Geometry: final body of the model. Coordinates: model frame, mm. Face numbers are marked on the shaded views. A direction names the side the tool comes from. Coordinates: 2 decimals unless noted, no trailing zeros. Write each loop counter-clockwise with the first axis right and the second up, starting at its lowest first coordinate (ties: lowest second). Pieces come first, ordered by that corner, then holes. Notation, with made-up numbers: (73, -15.5) -> (111, -15.5) arc R16 ccw to (111, 0.5) -> close; hole circle Ø6 at (37, -31.75). An arc over 180 degrees is marked (long way). One line per item, written item: value.
Autodesk Inventor part; units mm, degrees
ref_plane "Work Plane1" through (29, 0, 0) normal (0, -1, 0) x (1, 0, 0)
ref_plane "YZ Plane" through (0, 0, 0) normal (1, 0, 0) x (0, 1, 0)
ref_plane "XZ Plane" through (0, 0, 0) normal (0, 1, 0) x (-1, 0, 0)
sketch "Skizze1" plane through (0, 0, 0) normal (0, 0, 1) x (1, 0, 0)
  line L0 (-0.5, 0) -> (20, 0)
  line L1 (20, 0) -> (20, 1)
  line L2 (20, 1) -> (1, 1)
  line L3 (1, 1) -> (0.7545, 1)
  line L4 (0.7545, 1) -> (0, 1)
  line L5 (0, 1) -> (0, 1.9)
  line L6 (0, 1.9) -> (-2, 1.9)
  line L7 (-2, 1.9) -> (-2, 0.866)
  line L8 (-2, 0.866) -> (-1, 0.866)
  line L9 (-1, 0.866) -> (-0.5, 0)
  line L10 (-6.4, 0) -> (24.4, 0)
  line L11 (0, -0.38) -> (0, 2.28)
  line L12 (1, 1) -> (0, 1) construction
  dimension "d1" = 19
  dimension "d2" = 0.2455
  dimension "d3" = 2
  dimension "d4" = 1
  dimension "d5" = 60
  dimension "d6" = 2
  dimension "d7" = 2
  dimension "d8" = 1.7321
  dimension "d9" = 3.8
  dimension "d26" = 20
revolve "Körper" add sketch "Skizze1" angle 360 about axis through (-0.5, 0, 0) along (1, 0, 0)
sketch "Skizze2" plane through (-2, 0, 0) normal (-1, 0, 0) x (0, 0, 1)
  circle A0 centre (0, 0) radius 0.866
  line L0 (0, -2.66) -> (0, 2.66)
  line L1 (-2.66, 0) -> (2.66, 0)
  line L2 (0.866, 0) -> (0.433, -0.75)
  line L3 (0.433, -0.75) -> (-0.433, -0.75)
  line L4 (-0.433, -0.75) -> (-0.866, 0)
  line L5 (-0.866, 0) -> (-0.433, 0.75)
  line L6 (-0.433, 0.75) -> (0.433, 0.75)
  line L7 (0.433, 0.75) -> (0.866, 0)
extrude "Loch" add sketch "Skizze2" against normal up to next contours L7 A0 | A0 L2 | L6 L0 A0 | A0 L0 L3 | L0 L6 A0 | A0 L3 L0 | L4 A0 | A0 L5
fillet "Rundung1" radius 0.2 1 edges at (-2, -1.9, 0)
thread "Gewinde"
chamfer "Fase1" distance 0.2454 distance2 0.2454 1 edges at (20, -1, 0) measured on face at (20, -0.4443, -0.4503)
ref_plane "Work Plane1" through (29, 0, 0) normal (0, -1, 0) x (1, 0, 0)
fillet "Fillet2" radius 0.1 1 edges at (0, -1, 0)
equation "\"d1\" = GEL"
equation "\"d3\" = KOH"
equation "\"d4\" = INTI"
equation "\"d6\" = GD"
equation "\"d7\" = BDM"
equation "\"d8\" = 1.1547 * SW"
equation "\"d9\" = KOD"
equation "\"d26\" = NLG"
equation "\"d30\" = R"
equation "\"d17\" = RR"
equation "\"d13\" = GEL"
equation "\"d15\" = -0.5 * SPD + 0.5 * GD"
equation "\"d16\" = GUL"
equation "\"GD\" = NND"
equation "\"NLG\" = 20"
equation "\"GEL\" = 19"
equation "\"KOD\" = 3.8"
equation "\"KOH\" = 2"
equation "\"INTI\" = 1"
equation "\"GAL\" = 0.61345 * PTC"
equation "\"GUL\" = 0.61345 * PTC"
equation "\"BDM\" = NND"
equation "\"SW\" = 1.5"
equation "\"RR\" = 0.2"
equation "\"SPD\" = NND - 1.2269 * PTC"
equation "\"R\" = 0.1"
equation "\"TOA\" = 30deg"
equation "\"GD1\" = THREADDIA - 1.2269 * PTC"
equation "\"THREADDIA\" = 2"
equation "\"FAWI\" = 45deg"
equation "\"ANG\" = 120deg"
equation "\"PTC\" = 0.4"
equation "\"NND\" = 2"
equation "\"E0\" = 1.155 * SW"
properties part number "DIN 912 - M2 x 20" material "Stahl, weich"
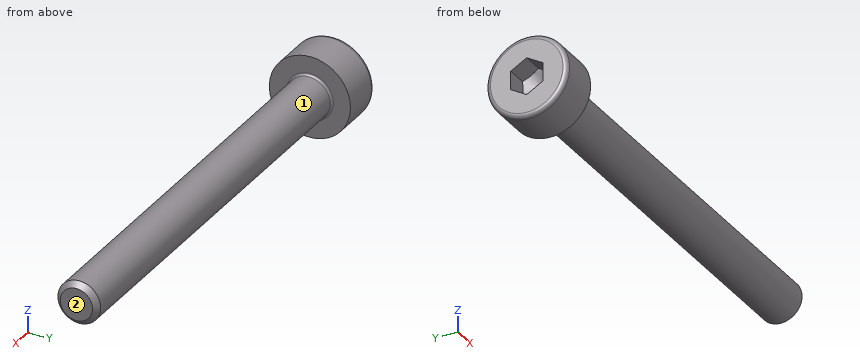
(1) First-contact query: pin 1 (2 mm diameter, centred on x = 13.5, z = -1.5, fed in from +Y); pin 2 (1 mm diameter, centred on x = 8, y = 0, fed in from +Z). Flat tips, straight axial feed; report the tip coordinate or a pass-through.
Responses:
pin 1: stops at y = 0.87
pin 2: stops at z = 1
(2) Section A-A (x = 7). Return the cut outline in (y, z).
Responses:
outline: circle Ø2 at (0, 0)
(3) Reachability of the marked faces 1 and 2 from +Z, -Z, +X, -X, +Y, -Y: full face, straight path, thin tool, end or side. Return the list, or none.
Responses:
face 1: +X
face 2: +Z, -Z, +X, +Y, -Y
(4) Line query: line 1 (X direction, y = 0.4, z = 1.3); line 2 (Z direction, x = 11.5, y = -0.1). Output: solid intervals per line, ascending. Write a range as [from, to].
Responses:
line 1: x = [-2, 0]
line 2: z = [-0.99, 0.99]
